Job drawing, mm, ordinate dimensions from the low corner. One solid piece. Coordinates: 2 decimals unless noted, no trailing zeros. Loops run counter-clockwise (first coordinate to the right, second up) from the corner with the lowest first, then second, coordinate; pieces in that order, holes last. Notation, with made-up numbers: (71, 66) -> (92, 66) arc R17 cw to (92, 83) -> close; hole circle Ø3 at (-3.75, 6). An arc over 180 degrees is marked (long way). Use one line per item in the form item = value. Start each with the question number.
(1) Drill centre lines: L1, parallel to X at y = 0.9, z = 80; L2, parallel to Z at x = 75, y = 1.2; L3, parallel to X at y = 1.4, z = 150. Where is each one in solid material? Low to high. Write a range as [from, to].
(2) Band-saw the part on A-A on z = 80. Give the cut face in (x, y).
(3) Pin check, flat tips, straight feed: P1, Ø1.5, axis at y = 1.5, z = 2, coming from the +X side; P2, Ø0.9, axis at y = 1.5, z = 16, coming from the +X side; P3, Ø0.9, axis at y = 2, z = 141.5, coming from the -X side. Stop position of each tip, or through.
(4) Band-saw the part on B-B on x = 75. Give the cut face in (y, z), then the cut area to 3 significant figures.
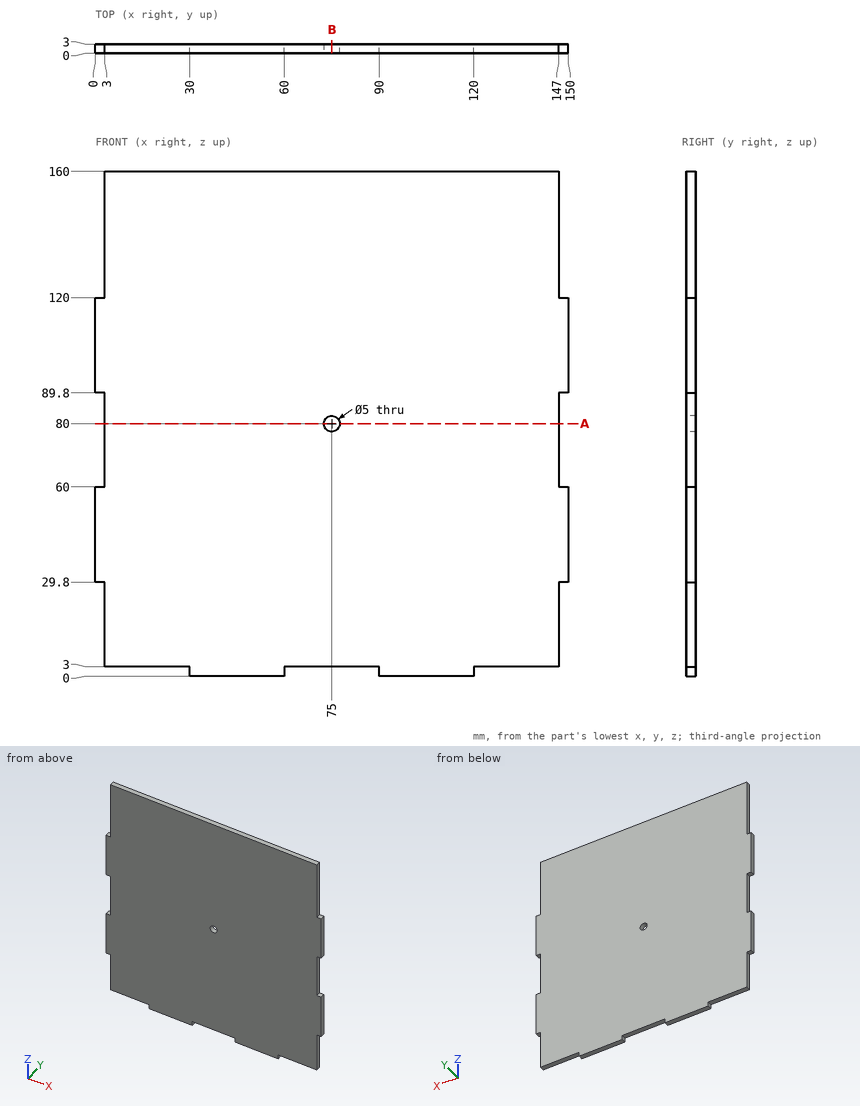
A:
q1.L1 = [3, 72.5], [77.5, 147]
q1.L2 = [3, 77.5], [82.5, 160]
q1.L3 = [3, 147]
q2.outline = (3, 0) -> (72.5, 0) -> (72.5, 3) -> (3, 3) -> close; (77.5, 0) -> (147, 0) -> (147, 3) -> (77.5, 3) -> close
q3.P1 = 120
q3.P2 = 147
q3.P3 = 3
q4.outline = (0, 3) -> (3, 3) -> (3, 77.5) -> (0, 77.5) -> close; (0, 82.5) -> (3, 82.5) -> (3, 160) -> (0, 160) -> close
q4.area = 456 mm²
